Can you work these out from the model? Positions are in its coordinate system, mm. Round coordinates to 2 decimals unless told otherwise and drop trailing zeros. Order: outer loops, then holes, each group sorted by start corner. A loop starts at its lowest first (then second) coordinate and runs counter-clockwise, first axis right, second up.
from build123d import *

# Parameters (mm, degrees)
SKETCH_1_W          = 12.6
SKETCH_1_H          = 12.6
EXTRUDE_1_DEPTH     = 22
CUT_EXTRUDE_1_REACH = 28.124
SKETCH_2_R          = 1.55
CUT_EXTRUDE_2_REACH = 28.124
SKETCH_3_R          = 1.55


with BuildPart() as part:
    # 草图1 → 凸台-拉伸1 (new body)
    with BuildSketch(Plane.XY):
        Rectangle(SKETCH_1_W, SKETCH_1_H)
    extrude(amount=EXTRUDE_1_DEPTH)

    # 草图2 → 切除-拉伸1 (cut, up to next)
    with BuildSketch(Plane(origin=(0, 6.3, 0), x_dir=(1, 0, 0), z_dir=(0, 1, 0)), mode=Mode.PRIVATE) as cut_extrude_1_sk1:
        with Locations(Location((0, -9, 0), (0, 0, 270))):
            Circle(SKETCH_2_R)
    cut_extrude_1_tool1 = extrude(cut_extrude_1_sk1.sketch, amount=-CUT_EXTRUDE_1_REACH, mode=Mode.PRIVATE) & part.part
    # 草图2 → 切除-拉伸1 (cut, up to next)
    with BuildSketch(Plane(origin=(0, 6.3, 0), x_dir=(1, 0, 0), z_dir=(0, 1, 0)), mode=Mode.PRIVATE) as cut_extrude_1_sk2:
        with Locations(Location((0, -16, 0), (0, 0, 270))):
            Circle(SKETCH_2_R)
    cut_extrude_1_tool2 = extrude(cut_extrude_1_sk2.sketch, amount=-CUT_EXTRUDE_1_REACH, mode=Mode.PRIVATE) & part.part
    add(cut_extrude_1_tool1.solids().sort_by_distance((0, 6.3, 9))[0], mode=Mode.SUBTRACT)
    add(cut_extrude_1_tool2.solids().sort_by_distance((0, 6.3, 16))[0], mode=Mode.SUBTRACT)

    # 切除-拉伸2: up to this face of the body (flat: up to its plane)
    cut_extrude_2_end = Plane(part.part.faces().sort_by_distance((6.3, 0, 11))[0])
    # 草图3 → 切除-拉伸2 (cut, up to the picked face)
    with BuildSketch(Plane.ZY.offset(6.3), mode=Mode.PRIVATE) as cut_extrude_2_sk1:
        with Locations((9, 0)):
            Circle(SKETCH_3_R)
    cut_extrude_2_tool1 = split(extrude(cut_extrude_2_sk1.sketch, amount=-CUT_EXTRUDE_2_REACH, mode=Mode.PRIVATE), bisect_by=cut_extrude_2_end, keep=Keep.BOTH, mode=Mode.PRIVATE)
    # 草图3 → 切除-拉伸2 (cut, up to the picked face)
    with BuildSketch(Plane.ZY.offset(6.3), mode=Mode.PRIVATE) as cut_extrude_2_sk2:
        with Locations((16, 0)):
            Circle(SKETCH_3_R)
    cut_extrude_2_tool2 = split(extrude(cut_extrude_2_sk2.sketch, amount=-CUT_EXTRUDE_2_REACH, mode=Mode.PRIVATE), bisect_by=cut_extrude_2_end, keep=Keep.BOTH, mode=Mode.PRIVATE)
    add(cut_extrude_2_tool1.solids().sort_by(Axis((-6.3, 0, 9), (1, 0, 0)))[0], mode=Mode.SUBTRACT)
    add(cut_extrude_2_tool2.solids().sort_by(Axis((-6.3, 0, 16), (1, 0, 0)))[0], mode=Mode.SUBTRACT)


solid = part.part
(1) I want a section at A-A, the plane y = 5.25. List the corners of the cut face in (x, z) for me, plus the area to 3 significant figures.
(2) I want a section at C-C, the plane x = -1. List the corners of the cut face in (y, z) for me.
(3) Please list where these lines run through material, in increasing order: probe 1 along X at (y, z) = (-3, 16); probe 2 along Z at (x, y) = (-3.5, -1).
(4) If we mould it in two halves opening along Y, with no side actions, what happens to faces 1 (the face through (0, 6.3, 11)), 2 (the face through (0, 0, 0)), 3 (the face through (0, -6.3, 11)), 4 (the face through (-3.89, 0.07, 7.45))? For each: pulls with the +Y half, pulls with the -Y half, needs draft (parallel to the pull), parting line crosses it, or undercut.
(5) I want a section at B-B, the plane z = 16. List the corners of the cut face in (x, y) for me.
(6) I'm going to push a flat-ended pin straight in: pin 1 Ø4 at (x, z) = (0, 16) entering from +Y. Where does the tip first touch, or does it pass through?
Ans:
1. outline: (-6.3, 0) - (6.3, 0) - (6.3, 22) - (-6.3, 22) - close; hole circle Ø3.1 at (0, 9); hole circle Ø3.1 at (0, 16)
1. area: 262 mm2
2. outline: (-6.3, 0) - (6.3, 0) - (6.3, 7.82) - (1, 7.82) arc R1.55 cw to (-1, 7.82) - (-6.3, 7.82) - close; (-6.3, 10.18) - (-1, 10.18) arc R1.55 cw to (1, 10.18) - (6.3, 10.18) - (6.3, 14.82) - (1, 14.82) arc R1.55 cw to (-1, 14.82) - (-6.3, 14.82) - close; (-6.3, 17.18) - (-1, 17.18) arc R1.55 cw to (1, 17.18) - (6.3, 17.18) - (6.3, 22) - (-6.3, 22) - close
3. probe 1: x = -6.3 to -1.55, 1.55 to 6.3
3. probe 2: z = 0 to 7.82, 10.18 to 14.82, 17.18 to 22
4. face 1: pulls with the +Y half
4. face 2: needs draft
4. face 3: pulls with the -Y half
4. face 4: undercut
5. outline: (-6.3, -6.3) - (-1.55, -6.3) - (-1.55, -1.55) - (-6.3, -1.55) - close; (-6.3, 1.55) - (-1.55, 1.55) - (-1.55, 6.3) - (-6.3, 6.3) - close; (1.55, -6.3) - (6.3, -6.3) - (6.3, -1.55) - (1.55, -1.55) - close; (1.55, 1.55) - (6.3, 1.55) - (6.3, 6.3) - (1.55, 6.3) - close
6. pin 1: stops at y = 6.3
